Solid Edge part; units mm, degrees
sketch "Sketch1" plane through (0, 0, 0) normal (0, 0, 1) x (1, 0, 0)
  line L0 (24.1, -18.75) -> (-24.1, -18.75)
  line L1 (-24.1, -18.75) -> (-24.1, 18.75)
  line L2 (-24.1, 18.75) -> (24.1, 18.75)
  line L3 (24.1, 18.75) -> (24.1, -18.75)
  dimension "D1" = 24.1
  dimension "D2" = 24.1
extrude "Protrusion1" add sketch "Sketch1" along normal blind 24.8
sketch "Sketch2" plane through (0, 0, 24.8) normal (0, 0, 1) x (1, 0, 0)
  line L0 (-20.9, 18.75) -> (20.9, 18.75)
  line L1 (20.9, 18.75) -> (20.9, -13.25)
  line L2 (20.9, -13.25) -> (-20.9, -13.25)
  line L3 (-20.9, -13.25) -> (-20.9, 18.75)
  dimension "D1" = 20.9
  dimension "D2" = 20.9
extrude "Cutout1" cut sketch "Sketch2" against normal through all
hole "Hole_1" at (-24.1, 7.75, 12.4) direction (1, 0, 0) diameter 8 depth 140
hole "Hole_2" at (-24.1, 15.75, 12.4) direction (1, 0, 0) diameter 2 end through all
hole "Hole1" at (-24.1, 7.75, 20.4) direction (1, 0, 0) diameter 2 end through all
hole "Hole2" at (-24.1, -0.25, 12.4) direction (1, 0, 0) diameter 2 end through all
hole "Hole3" at (-24.1, 7.75, 4.4) direction (1, 0, 0) diameter 2 end through all
hole "Hole_6" at (-24.1, -8.25, 20.4) direction (1, 0, 0) diameter 1.7 end through all
hole "Hole4" at (-24.1, -8.25, 4.4) direction (1, 0, 0) diameter 1.7 end through all
fillet "Round_1" radius 12.4 4 edges at (-22.5, 18.75, 24.8) (-22.5, 18.75, 0) (22.5, 18.75, 24.8) (22.5, 18.75, 0)
hole "Hole_8" at (0, -18.75, 20.8028) direction (0, 1, 0) diameter 2 end through all
hole "Hole5" at (0, -18.75, 4.8795) direction (0, 1, 0) diameter 2 end through all
hole "Hole6" at (8, -18.75, 4.8795) direction (0, 1, 0) diameter 2 end through all
hole "Hole7" at (8, -18.75, 12.4) direction (0, 1, 0) diameter 2 end through all
hole "Hole8" at (8, -18.75, 20.8028) direction (0, 1, 0) diameter 2 end through all
hole "Hole9" at (16, -18.75, 20.8028) direction (0, 1, 0) diameter 2 end through all
hole "Hole10" at (16, -18.75, 4.8795) direction (0, 1, 0) diameter 2 end through all
hole "Hole11" at (-8, -18.75, 20.8028) direction (0, 1, 0) diameter 2 end through all
hole "Hole12" at (-8, -18.75, 12.4) direction (0, 1, 0) diameter 2 end through all
hole "Hole13" at (-8, -18.75, 4.8795) direction (0, 1, 0) diameter 2 end through all
hole "Hole14" at (-16, -18.75, 4.8795) direction (0, 1, 0) diameter 2 end through all
hole "Hole15" at (-16, -18.75, 20.8028) direction (0, 1, 0) diameter 2 end through all
CAD build for the part. Positions are in the model's coordinates, mm. Coordinates: 2 decimals unless noted, no trailing zeros. Loops run counter-clockwise (first coordinate to the right, second up) from the corner with the lowest first, then second, coordinate; pieces in that order, holes last. Notation, with made-up numbers: (-13.75, -34) - (37.25, -34) arc R19 ccw to (37.25, -16) - close; hole circle Ø10 at (-2.5, 18). An arc over 180 degrees is marked (long way). Return JSON: item names as keys, results as strings.
1. Band-saw the part on A-A (x = -16). Give the cut face in (y, z).
Result:
{"outline": "(-18.75, 0) - (-13.25, 0) - (-13.25, 3.88) - (-18.75, 3.88) - close; (-18.75, 5.88) - (-13.25, 5.88) - (-13.25, 19.8) - (-18.75, 19.8) - close; (-18.75, 21.8) - (-13.25, 21.8) - (-13.25, 24.8) - (-18.75, 24.8) - close"}
2. Band-saw the part on C-C (y = -2). Give the cut face in (x, z).
Result:
{"outline": "(-24.1, 0) - (-20.9, 0) - (-20.9, 24.8) - (-24.1, 24.8) - close; (20.9, 0) - (24.1, 0) - (24.1, 24.8) - (20.9, 24.8) - close"}
3. Band-saw the part on D-D (x = -8). Give the cut face in (y, z).
Result:
{"outline": "(-18.75, 0) - (-13.25, 0) - (-13.25, 3.88) - (-18.75, 3.88) - close; (-18.75, 5.88) - (-13.25, 5.88) - (-13.25, 11.4) - (-18.75, 11.4) - close; (-18.75, 13.4) - (-13.25, 13.4) - (-13.25, 19.8) - (-18.75, 19.8) - close; (-18.75, 21.8) - (-13.25, 21.8) - (-13.25, 24.8) - (-18.75, 24.8) - close"}
4. Drop flat-ended pins along their axis: pin 1 (1.6 mm diameter, centred on x = -16, z = 4.88, fed in from +Y); pin 2 (10 mm diameter, centred on x = 11, z = 11.5, fed in from +Y). Give the stop position or say it passes through.
Result:
{"pin 1": "passes through", "pin 2": "stops at y = -13.25"}
5. Band-saw the part on B-B (y = -8.25). Give the cut face in (x, z), and give its area (3 significant figures).
Result:
{"outline": "(-24.1, 0) - (-20.9, 0) - (-20.9, 3.55) - (-24.1, 3.55) - close; (-24.1, 5.25) - (-20.9, 5.25) - (-20.9, 19.55) - (-24.1, 19.55) - close; (-24.1, 21.25) - (-20.9, 21.25) - (-20.9, 24.8) - (-24.1, 24.8) - close; (20.9, 0) - (24.1, 0) - (24.1, 3.55) - (20.9, 3.55) - close; (20.9, 5.25) - (24.1, 5.25) - (24.1, 19.55) - (20.9, 19.55) - close; (20.9, 21.25) - (24.1, 21.25) - (24.1, 24.8) - (20.9, 24.8) - close", "area": "137 mm2"}
6. Mould opens along Y. For faces 1 (the flat face through (0, -18.75, 12)), 2 (the flat face through (24.1, -4, 12)), 3 (the cylindrical face through (22.5, -0.2, 11.4)) say: released by +Y, released by -Y, zero draft, split by the parting line, or undercut.
Result:
{"face 1": "released by -Y", "face 2": "zero draft", "face 3": "undercut"}
7. Probe L1, parallel to Y at x = -23, z = 12.4; L2, parallel to Z at x = 8, y = -17; L3, parallel to X at y = -8, z = 9.25. List the from-to ranges inside material, lowest first. Write a range as from..to.
Result:
{"L1": "y = -18.75..-1.25, 0.75..3.75, 11.75..14.75, 16.75..18.75", "L2": "z = 0..3.88, 5.88..11.4, 13.4..19.8, 21.8..24.8", "L3": "x = -24.1..-20.9, 20.9..24.1"}
